```python
from build123d import *

# Parameters (mm, degrees)
F0_W      = 96
F0_H      = 64
F1_DEPTH  = 16
F3_DEPTH  = 16
F5_DEPTH  = 16
F6_W      = 40
F6_H      = 28
F7_DEPTH  = 42
F9_DEPTH  = 42
F11_DEPTH = 12


with BuildPart() as f1:
    # F0 (on Top) → F1 (new body)
    with BuildSketch(Plane.XY):
        with Locations((-6.250218, 25.54076)):
            Rectangle(F0_W, F0_H)
    extrude(amount=F1_DEPTH)

    # F2 (on face) → F3 (join)
    with BuildSketch(Plane(origin=(-54.250218, 0, 0), x_dir=(0, -1, 0), z_dir=(-1, 0, 0))):
        with BuildLine():
            Line((-57.54076, 16), (6.45924, 16))
            Line((6.45924, 16), (6.45924, 44))
            ThreePointArc((6.45924, 44), (-5.31701, 58.532998), (-23.205554, 64))
            Line((-23.205554, 64), (-57.54076, 64))
            Line((-57.54076, 64), (-57.54076, 16))
        make_face()
    extrude(amount=-F3_DEPTH)

    # F4 (on face) → F5 (cut)
    with BuildSketch(Plane.XY.offset(16)):
        with BuildLine():
            Line((21.749782, 9.54076), (41.749782, 9.54076))
            Line((41.749782, 9.54076), (41.749782, 25.54076))
            Line((41.749782, 25.54076), (21.749782, 25.54076))
            ThreePointArc((21.749782, 25.54076), (13.749782, 17.54076), (21.749782, 9.54076))
        make_face()
    extrude(amount=-F5_DEPTH, mode=Mode.SUBTRACT)

    # F6 (on face) → F7 (join)
    with BuildSketch(Plane(origin=(0, 57.54076, 0), x_dir=(-1, 0, 0), z_dir=(0, 1, 0))):
        with Locations((18.250218, 30)):
            Rectangle(F6_W, F6_H)
    extrude(amount=-F7_DEPTH)

    # F8 (on face) → F9 (cut)
    with BuildSketch(Plane(origin=(0, 57.54076, 0), x_dir=(-1, 0, 0), z_dir=(0, 1, 0))):
        with BuildLine():
            ThreePointArc((6.250218, 44), (18.250218, 32), (30.250218, 44))
            Line((30.250218, 44), (6.250218, 44))
        make_face()
    extrude(amount=-F9_DEPTH, mode=Mode.SUBTRACT)

    # F10 (on face) → F11 (join)
    with BuildSketch(Plane(origin=(0, 57.54076, 0), x_dir=(-1, 0, 0), z_dir=(0, 1, 0))):
        Polygon((-41.749782, 16), (-1.749782, 16), (-1.749782, 44), align=None)
    extrude(amount=-F11_DEPTH)


solid = f1.part
```
The listing builds one solid part. Answer for the finished solid, in the listing's coordinates (mm). A direction names the side the tool comes from. Give positions to 0.01 mm unless a question says otherwise; leave off trailing zeros. Write each loop counter-clockwise with the first axis right and the second up, starting at its lowest first coordinate (ties: lowest second). Pieces come first, ordered by that corner, then holes. Notation, with made-up numbers: (31, -33) -> (44, -33) arc R21 cw to (44, 4) -> close; hole circle Ø3 at (-15, 43.25). An arc over 180 degrees is marked (long way). Use one line per item in the form item = value.
1) Section D-D on x = -36.5 is taken. Write down the section's boundary in (y, z).
Result:
outline = (-6.46, 0) -> (57.54, 0) -> (57.54, 44) -> (15.54, 44) -> (15.54, 16) -> (-6.46, 16) -> close
2) Straight lines are drawn through the part: probe 1 along X at (y, z) = (55.5, 48); probe 2 along X at (y, z) = (24.5, 35); probe 3 along Y at (x, z) = (9.5, 19.5). For each, find the intervals that lie inside material, in ascending order.
Result:
probe_1 = -54.25 to -38.25
probe_2 = -54.25 to -26.19, -10.31 to 1.75
probe_3 = 45.54 to 57.54
3) For a pull along Y with two mould halves and no side action, classify faces 5 (the cylindrical face through (13.75, 17.72, 8.11)), 6 (the flat face through (10, 14, 16)), 7 (the flat face through (13, 45.541, 24)) as +Y half, -Y half, draft (parallel to the pull), parting line (faces both ways), or undercut.
Result:
face_5 = undercut
face_6 = draft
face_7 = -Y half
4) A tool of negligible diameter and unlimited length cuts with its end or side. For faces 1 (the flat face through (1.75, 31, 30)), 2 (the flat face through (-2, 37, 44)), 3 (the flat face through (32, 9.541, 8)), 4 (the flat face through (41.75, 1, 8)), from which of +Z, -Z, +X, -X, +Y, -Y can it reach the whole face along a straight path? Write none if from no direction.
Result:
face_1 = +Z, +X, -Y
face_2 = +Z, +X, +Y, -Y
face_3 = +Z, -Z, +X
face_4 = +Z, -Z, +X, +Y, -Y
5) Section B-B on x = 27.5 is taken. Write down the section's boundary in (y, z).
Result:
outline = (-6.46, 0) -> (9.54, 0) -> (9.54, 16) -> (-6.46, 16) -> close; (25.54, 0) -> (57.54, 0) -> (57.54, 25.97) -> (45.54, 25.97) -> (45.54, 16) -> (25.54, 16) -> close
6) Section C-C on z = 35 is taken. Write down the section's boundary in (x, y).
Result:
outline = (-54.25, -6.46) -> (-38.25, -6.46) -> (-38.25, 15.54) -> (-26.19, 15.54) -> (-26.19, 57.54) -> (-54.25, 57.54) -> close; (-10.31, 15.54) -> (1.75, 15.54) -> (1.75, 45.54) -> (14.61, 45.54) -> (14.61, 57.54) -> (-10.31, 57.54) -> close
7) Section A-A on y = 38 is taken. Write down the section's boundary in (x, z), plus the area to 3 significant figures.
Result:
outline = (-54.25, 0) -> (41.75, 0) -> (41.75, 16) -> (1.75, 16) -> (1.75, 44) -> (-6.25, 44) arc R12 cw to (-30.25, 44) -> (-38.25, 44) -> (-38.25, 64) -> (-54.25, 64) -> close
area = 3,200 mm²
8) Each of these flat-tipped pins is pushed along its axis until it touches: P1, Ø8.5, axis at x = 24, z = 30.5, coming from the -Y side; P2, Ø8.5, axis at y = 33, z = 36, coming from the +X side; P3, Ø1.5, axis at x = 21.5, y = 38.5, coming from the +Z side; P4, Ø22.5, axis at x = -12, z = 26.5, coming from the -Y side. Where does it stop, or does it pass through?
Result:
P1 = 45.54
P2 = 1.75
P3 = 16
P4 = -6.46
